Design review of the part built by this model. Coordinates are the model's own, in mm. Give positions to 0.01 mm unless a question says otherwise; leave off trailing zeros. Loops run counter-clockwise (first coordinate to the right, second up) from the corner with the lowest first, then second, coordinate; pieces in that order, holes last. Notation, with made-up numbers: (1.25, -25) - (20.25, -25) arc R15 cw to (20.25, -20) - close; hole circle Ø5 at (74.5, 76). An arc over 180 degrees is marked (long way). Write each question's results on one line, items separated by ' | '.
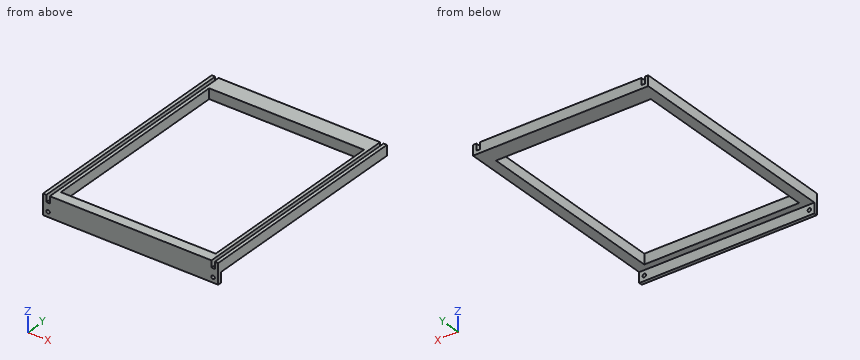
```python
from build123d import *

# Parameters (mm, degrees)
F0_W     = 516
F0_H     = 660
F0_W_2   = 456
F0_H_2   = 580
F1_DEPTH = 20
F2_W     = 10
F2_H     = 660
F3_DEPTH = 10
F4_DEPTH = 10
F5_W     = 30
F5_H     = 10
F6_DEPTH = 30
F8_D     = 10
F9_DEPTH = 456


with BuildPart() as f1:
    # F0 (on Top) → F1 (new body)
    with BuildSketch(Plane.XY):
        with Locations((30.9582352638, 132.1864551082)):
            Rectangle(F0_W, F0_H)
        with Locations((30.9582352638, 122.1864551082)):
            Rectangle(F0_W_2, F0_H_2, mode=Mode.SUBTRACT)
    extrude(amount=F1_DEPTH)

    # F2 (on face) → F3 (cut)
    with BuildSketch(Plane.XY.offset(20)):
        with Locations((-212.0417647362, 132.1864551082)):
            Rectangle(F2_W, F2_H)
        with Locations((273.9582352638, 132.1864551082)):
            Rectangle(F2_W, F2_H)
    extrude(amount=-F3_DEPTH, mode=Mode.SUBTRACT)

    # F4 (add): faces of the model
    f4_faces = [f1.faces().sort_by_distance(p)[0] for p in [
        (283.9582352638, 132.1864551082, 20),
        (-222.0417647362, 132.1864551082, 20),
        (30.9582352638, -189.6761251533, 20),
    ]]
    extrude(f4_faces, amount=F4_DEPTH)

    # F5 (on face) → F6 (join)
    with BuildSketch(Plane(origin=(0, 0, 0), x_dir=(1, 0, 0), z_dir=(0, 0, -1))):
        with Locations((273.9582352638, 192.8135448918)):
            Rectangle(F5_W, F5_H)
        with Locations((-212.0417647362, 192.8135448918)):
            Rectangle(F5_W, F5_H)
    extrude(amount=F6_DEPTH)

    # F8 (through all)
    with Locations(Plane(origin=(0, -187.8135448918, 0), x_dir=(-1, 0, 0), z_dir=(0, 1, 0))):
        with Locations((212.0417647362, -15), (-273.9582352638, -15)):
            Hole(F8_D / 2)

    # F9 (add, through all): a face of the model
    f9_faces = [f1.faces().sort_by_distance(p)[0] for p in [
        (258.9582352638, -192.8135448918, -15),
    ]]
    extrude(f9_faces, amount=F9_DEPTH)


solid = f1.part
```
Item 1: We need section B-B on x = -23. Give the boundary of the cut face in (y, z), then the cut area to 3 significant figures.
Output values:
outline: (-197.81, -30) - (-187.81, -30) - (-187.81, 0) - (-167.81, 0) - (-167.81, 30) - (-197.81, 30) - close; (412.19, 0) - (462.19, 0) - (462.19, 30) - (412.19, 30) - close | area: 2,700 mm²
Item 2: Wall thickness on probe 1 along X at (y, z) = (385, 18); probe 2 along Y at (x, z) = (-96.5, 12.5); probe 3 along X at (y, z) = (106, 0.5): over which ranges is each line inside the solid? List them lowest first.
Output values:
probe 1: x = -227.04 to -217.04, -207.04 to -197.04, 258.96 to 268.96, 278.96 to 288.96 | probe 2: y = -197.81 to -167.81, 412.19 to 462.19 | probe 3: x = -227.04 to -197.04, 258.96 to 288.96
Item 3: We need section A-A on y = 224.5. Give the boundary of the cut face in (x, z), then the cut area to 3 significant figures.
Output values:
outline: (-227.04, 0) - (-197.04, 0) - (-197.04, 30) - (-207.04, 30) - (-207.04, 10) - (-217.04, 10) - (-217.04, 30) - (-227.04, 30) - close; (258.96, 0) - (288.96, 0) - (288.96, 30) - (278.96, 30) - (278.96, 10) - (268.96, 10) - (268.96, 30) - (258.96, 30) - close | area: 1,400 mm²
Item 4: Clearance check with flat-ended pins moving along their axes: P1, Ø9, axis at x = 113, z = -8, coming from the +Y side; P2, Ø3, axis at x = -210, y = 208.5, coming from the +Z side. State where each tip first meets the part, or that it passes through.
Output values:
P1: stops at y = -187.81 | P2: stops at z = 10
